from build123d import *

# Parameters (mm, degrees)
SKETCH037_R     = 5
SKETCH037_R_2   = 3
PAD019_DEPTH    = 7
PAD020_DEPTH    = 50
POCKET019_DEPTH = 52
SKETCH055_W     = 120.3
SKETCH055_H     = 69.7
POCKET033_DEPTH = 2


with BuildPart() as part:
    # Sketch037 → Pad019 (new body)
    with BuildSketch(Plane.XZ):
        with BuildLine():
            Line((-74.137414, 12.904758), (-74.137414, 35.098297))
            Line((-81.471367, 35.098297), (-74.137414, 35.098297))
            ThreePointArc((-86.471367, 40.098297), (-85.006901, 36.562763), (-81.471367, 35.098297))
            Line((-86.471367, 91.234717), (-86.471367, 40.098297))
            ThreePointArc((-86.471367, 91.234717), (-60.36938, 92.892964), (-34.688969, 97.850786))
            ThreePointArc((34.688969, 97.850786), (0, 104.060193), (-34.688969, 97.850786))
            ThreePointArc((34.688969, 97.850786), (60.36938, 92.892964), (86.471367, 91.234717))
            Line((86.471367, 40.098297), (86.471367, 91.234717))
            ThreePointArc((81.471367, 35.098297), (85.006901, 36.562763), (86.471367, 40.098297))
            Line((81.471367, 35.098297), (74.137414, 35.098297))
            Line((74.137414, 35.098297), (74.137414, 12.904758))
            ThreePointArc((66.272551, 5.039896), (71.833849, 7.343461), (74.137414, 12.904758))
            Line((-66.272551, 5.039896), (66.272551, 5.039896))
            ThreePointArc((-74.137414, 12.904758), (-71.833849, 7.343461), (-66.272551, 5.039896))
        make_face()
        with Locations((50, 14)):
            Circle(SKETCH037_R, mode=Mode.SUBTRACT)
        with Locations((28, 14)):
            Circle(SKETCH037_R_2, mode=Mode.SUBTRACT)
        with Locations((-28, 14)):
            Circle(SKETCH037_R_2, mode=Mode.SUBTRACT)
        with Locations((-50, 14)):
            Circle(SKETCH037_R, mode=Mode.SUBTRACT)
    extrude(amount=PAD019_DEPTH)

    # Sketch038 → Pad020 (join)
    with BuildSketch(Plane.XZ):
        with BuildLine():
            ThreePointArc((-86.959112, 90.862971), (-61.522638, 92.265374), (-36.457272, 96.816017))
            ThreePointArc((36.457272, 96.816017), (0, 103.814452), (-36.457272, 96.816017))
            ThreePointArc((36.457272, 96.816017), (61.522638, 92.265374), (86.959112, 90.862971))
            Line((86.959112, 90.862971), (86.959112, 41.431149))
            ThreePointArc((80.824745, 35.296782), (85.162398, 37.093496), (86.959112, 41.431149))
            Line((80.824745, 35.296782), (73.659845, 35.296782))
            Line((73.659845, 35.296782), (73.659845, 29.983299))
            ThreePointArc((35.609044, 40.041003), (54.393041, 34.09886), (73.659845, 29.983299))
            ThreePointArc((35.609044, 40.041003), (0, 46.461552), (-35.609044, 40.041003))
            ThreePointArc((-73.659845, 29.983299), (-54.392205, 34.095699), (-35.609044, 40.041003))
            Line((-73.659845, 35.296782), (-73.659845, 29.983299))
            Line((-73.659845, 35.296782), (-80.824745, 35.296782))
            ThreePointArc((-86.959112, 41.431149), (-85.162398, 37.093496), (-80.824745, 35.296782))
            Line((-86.959112, 41.431149), (-86.959112, 90.862971))
        make_face()
    extrude(amount=-PAD020_DEPTH)

    # Sketch041 → Pocket019 (cut)
    with BuildSketch(Plane.XZ.offset(7)):
        with BuildLine():
            Line((-82.380554, 87.705044), (-82.380554, 41.80913))
            Line((-82.380554, 41.80913), (-70.96716, 41.80913))
            Line((-70.96716, 41.80913), (-70.96716, 33.384282))
            ThreePointArc((-70.96716, 33.384282), (-53.906892, 37.605949), (-37.282812, 43.308157))
            ThreePointArc((37.282812, 43.308157), (0, 50.369381), (-37.282812, 43.308157))
            ThreePointArc((37.282812, 43.308157), (53.912566, 37.625207), (70.96716, 33.384282))
            Line((70.96716, 41.80913), (70.96716, 33.384282))
            Line((82.380554, 41.80913), (70.96716, 41.80913))
            Line((82.380554, 87.705044), (82.380554, 41.80913))
            ThreePointArc((26.263667, 95.117414), (54.064692, 89.462391), (82.380554, 87.705044))
            ThreePointArc((26.263667, 95.117414), (0, 98.684945), (-26.263667, 95.117414))
            ThreePointArc((-82.380554, 87.705044), (-54.064692, 89.462391), (-26.263667, 95.117414))
        make_face()
    extrude(amount=-POCKET019_DEPTH, mode=Mode.SUBTRACT)

    # Sketch055 → Pocket033 (cut)
    with BuildSketch(Plane(origin=(6, -7, 41), x_dir=(1, 0, 0), z_dir=(0, -1, 0))):
        with Locations((-3.04, -0.08)):
            Rectangle(SKETCH055_W, SKETCH055_H)
    extrude(amount=-POCKET033_DEPTH, mode=Mode.SUBTRACT)


solid = part.part
Build history of the part. All positions in model axes, mm. A direction names the side the tool comes from. Round coordinates to 2 decimals unless told otherwise and drop trailing zeros. Order: outer loops, then holes, each group sorted by start corner. A loop starts at its lowest first (then second) coordinate and runs counter-clockwise, first axis right, second up. Notation, with made-up numbers: M 35,65.25 L 61,65.25 A32 cw 61,96.25 Z; hole C -4,-8 d6. An arc over 180 degrees is marked long. Use CSV: the item, a comma, the result in double quotes. Start each with the question number.
(1) Cut at B-B on y = 24.5. List the corners of the cut face in (x, z), then the cut area to 3 significant figures.
(2) Flat gauge pins, fed straight in: P1, Ø5.5, axis at x = -28, z = 14, coming from the +Y side; P2, Ø1, axis at x = -49.5, y = 34.5, coming from the -Z side; P3, Ø4, axis at y = 14, z = 38, coming from the +X side; P4, Ø1.6, axis at y = -6, z = 16.5, coming from the +X side. Where does each tip first touch, or does it go through?
(3) Drill centre lines: probe 1 along X at (y, z) = (-3, 14); probe 2 along X at (y, z) = (32, 55); probe 3 along Z at (x, y) = (50, -2). Where is each one in solid material? Low to high.
(4) Cut at D-D on x = 28. List the corners of the cut face in (y, z).
(5) Cut at A-A on z = 76. List the corners of the cut face in (x, y).
(6) Tool access for faces 1 (the face through (0.53, 19.65, 50.37)), 2 (the face through (-86.471, -3, 66)), 3 (the face through (78, -3, 35.098)), 4 (the face through (-85.21, 24.65, 37.14)): list every direction of +Z, -Z, +X, -X, +Y, -Y with a clear straight run to the whole face (end or side of a thin tool).
(7) Cut at C-C on x = -76. List the corners of the cut face in (y, z).
Findings:
1,outline,"M -86.96,41.43 A6.13 ccw -80.82,35.3 L -73.66,35.3 L -73.66,29.98 A204.74 ccw -35.61,40.04 A101.96 cw 35.61,40.04 A205.44 ccw 73.66,29.98 L 73.66,35.3 L 80.82,35.3 A6.13 ccw 86.96,41.43 L 86.96,90.86 A204.72 cw 36.46,96.82 A98.46 ccw -36.46,96.82 A204.72 cw -86.96,90.86 Z; hole M -82.38,41.81 L -70.97,41.81 L -70.97,33.38 A200.12 ccw -37.28,43.31 A101.96 cw 37.28,43.31 A205.44 ccw 70.97,33.38 L 70.97,41.81 L 82.38,41.81 L 82.38,87.71 A204.72 cw 26.26,95.12 A98.46 ccw -26.26,95.12 A204.72 cw -82.38,87.71 Z"
1,area,"1,900 mm^2"
2,P1,"passes through"
2,P2,"stops at z = 35.31"
2,P3,"stops at x = 86.79"
2,P4,"stops at x = 74.14"
3,probe 1,"x = -74.14 to -55, -45 to -31, -25 to 25, 31 to 45, 55 to 74.14"
3,probe 2,"x = -86.96 to -82.38, 82.38 to 86.96"
3,probe 3,"z = 5.04 to 9, 19 to 38.82, 90.04 to 94.49"
4,outline,"M -7,5.04 L 0,5.04 L 0,11 L -5,11 L -5,6.07 L -7,6.07 Z; M -7,94.65 L 45,94.65 L 45,46.45 L -5,46.45 L -5,17 L 0,17 L 0,42.54 L 50,42.54 L 50,99.75 L 0,99.75 L 0,100.06 L -7,100.06 Z"
5,outline,"M -86.96,0 L -86.47,0 L -86.47,-7 L -82.38,-7 L -82.38,45 L 82.38,45 L 82.38,-7 L 86.47,-7 L 86.47,0 L 86.96,0 L 86.96,50 L -86.96,50 Z"
6,face 1,"-Y"
6,face 2,"+Z, -Z, -X, -Y"
6,face 3,"-Z, +X, +Y, -Y"
6,face 4,"-Z, -X, +Y"
7,outline,"M -7,35.1 L 0,35.1 L 0,35.3 L 50,35.3 L 50,91.08 L 0,91.08 L 0,91.5 L -7,91.5 L -7,87.76 L 45,87.76 L 45,41.81 L -7,41.81 Z"
